Geometry: final body of the model. Coordinates: model frame, mm. A direction names the side the tool comes from. Give positions to 0.01 mm unless a question says otherwise; leave off trailing zeros. Order: outer loops, then holes, each group sorted by start corner. A loop starts at its lowest first (then second) coordinate and runs counter-clockwise, first axis right, second up. Notation, with made-up numbers: (40.5, -29) -> (69.5, -29) arc R11 cw to (69.5, -9) -> close; hole circle Ø1 at (38, -12). An arc over 180 degrees is marked (long way). One line per question, with ' | ' between items.
from build123d import *

# Parameters (mm, degrees)
SKETCH1_W             = 241.3
SKETCH1_H             = 50.8
BOSS_EXTRUDE1_DEPTH   = 12.7
SKETCH3_R             = 4
CUT_EXTRUDE1_DEPTH    = 124.947055229
CUT_EXTRUDE2_DEPTH    = 124.947055229
F_8_CLEARANCE_HOLE1_D = 4.4958
SKETCH10_R            = 1.905
CUT_EXTRUDE3_DEPTH    = 5.08
BOSS_EXTRUDE2_DEPTH   = 12.7
CUT_EXTRUDE4_DEPTH    = 124.947055239
SKETCH14_R            = 1.27
CUT_EXTRUDE5_DEPTH    = 6.35
SKETCH15_W            = 7.607640742
SKETCH15_H            = 9.409671306
CUT_EXTRUDE6_DEPTH    = 124.947055239
SKETCH16_W            = 0.104572849
SKETCH16_H            = 0.14582332
CUT_EXTRUDE8_DEPTH    = 124.947055239
SKETCH18_R            = 2.0828
CUT_EXTRUDE9_DEPTH    = 132.523201385
LPATTERN1_COUNT       = 3
LPATTERN1_PITCH       = 10.16


with BuildPart() as part:
    # Sketch1 → Boss-Extrude1 (new body)
    with BuildSketch(Plane.XY):
        Rectangle(SKETCH1_W, SKETCH1_H)
    extrude(amount=BOSS_EXTRUDE1_DEPTH)

    # Sketch3 → Cut-Extrude1 (cut, through all)
    with BuildSketch(Plane.XY.offset(12.7)):
        with Locations((-107.95, 0)):
            Circle(SKETCH3_R)
    extrude(amount=-CUT_EXTRUDE1_DEPTH, mode=Mode.SUBTRACT)

    # Sketch5 → Cut-Extrude2 (cut, through all)
    with BuildSketch(Plane.XY.offset(12.7)):
        with BuildLine():
            Line((-59.990308431, -25.4), (-105.894198974, -6.008009832))
            Line((-105.894198974, -6.008009832), (-109.958209517, -6.024084539))
            Line((-109.958209517, -6.024084539), (-118.086209517, -6.024084539))
            Line((-118.086209517, -6.024084539), (-118.086209517, 2.230915461))
            Line((-118.086209517, 2.230915461), (-113.895209517, 2.230915461))
            ThreePointArc((-113.895209517, 2.230915461), (-111.566364668, 5.219617475), (-107.95, 6.35))
            Line((-107.95, 6.35), (-67.015128773, 25.4))
            Line((-67.015128773, 25.4), (-120.65, 25.4))
            Line((-120.65, 25.4), (-120.65, -25.4))
            Line((-120.65, -25.4), (-59.990308431, -25.4))
        make_face()
        with BuildLine():
            Line((120.65, -25.4), (120.65, 25.4))
            ThreePointArc((120.65, 25.4), (72.371753541, -10.785174559), (13.834903468, -25.4))
            Line((13.834903468, -25.4), (120.65, -25.4))
        make_face()
    extrude(amount=-CUT_EXTRUDE2_DEPTH, mode=Mode.SUBTRACT)

    # #8 Clearance Hole1 (through all)
    with Locations(Plane(origin=(0, 0, 0), x_dir=(-1, 0, 0), z_dir=(0, 0, -1))):
        with Locations((44.020428639, 16.052306877), (44.020428639, -2.997693123)):
            f_8_clearance_hole1 = Hole(F_8_CLEARANCE_HOLE1_D / 2)

    # Sketch10 → Cut-Extrude3 (cut)
    with BuildSketch(Plane.ZY.offset(114.3)):
        with Locations((6.089367744, 0)):
            Circle(SKETCH10_R)
    extrude(amount=-CUT_EXTRUDE3_DEPTH, mode=Mode.SUBTRACT)

    # Sketch11 → Boss-Extrude2 (add)
    with BuildSketch(Plane.XY.offset(12.7)):
        Polygon((-93.824923554, 12.923434781), (-109.445923554, 5.653836977), (-109.445923554, 11.556774368), align=None)
    extrude(amount=-BOSS_EXTRUDE2_DEPTH)

    # Sketch12 → Cut-Extrude4 (cut, through all)
    with BuildSketch(Plane.XY.offset(12.7)):
        with BuildLine():
            Line((10.021655843, 16.51), (-33.573281826, 16.51))
            Line((-33.573281826, 16.51), (-33.573281826, -16.51))
            Line((-33.573281826, -16.51), (13.63000586, -16.51))
            ThreePointArc((13.63000586, -16.51), (23.12933387, -15.748429471), (32.557173193, -14.358081305))
            Line((32.557173193, -14.358081305), (10.021655843, 16.51))
        make_face()
        with BuildLine():
            Line((26.733875346, 16.51), (46.823064271, -11.007216822))
            ThreePointArc((46.823064271, -11.007216822), (74.177600846, 0.070720235), (98.687628211, 16.51))
            Line((98.687628211, 16.51), (26.733875346, 16.51))
        make_face()
    extrude(amount=-CUT_EXTRUDE4_DEPTH, mode=Mode.SUBTRACT)

    # Sketch14 → Cut-Extrude5 (cut)
    with BuildSketch(Plane(origin=(0.022106899, -5.589070571, 0), x_dir=(0.9999921775754317, 0.003955349282477503, 0), z_dir=(0.003955349282477503, -0.9999921775754317, 0))):
        with Locations((-107.949155569, 6.35)):
            Circle(SKETCH14_R)
    extrude(amount=-CUT_EXTRUDE5_DEPTH, mode=Mode.SUBTRACT)

    # Sketch15 → Cut-Extrude6 (cut, through all)
    with BuildSketch(Plane.XY.offset(12.7)):
        with Locations((113.836536756, 17.520164347)):
            Rectangle(SKETCH15_W, SKETCH15_H)
    extrude(amount=-CUT_EXTRUDE6_DEPTH, mode=Mode.SUBTRACT)

    # Sketch16 → Cut-Extrude8 (cut, through all)
    with BuildSketch(Plane.XY.offset(12.7)):
        with Locations((117.692643551, 22.15208834)):
            Rectangle(SKETCH16_W, SKETCH16_H)
    extrude(amount=-CUT_EXTRUDE8_DEPTH, mode=Mode.SUBTRACT)

    # Sketch18 → Cut-Extrude9 (cut, through all)
    with BuildSketch(Plane(origin=(0, 25.4, 0), x_dir=(1, 0, 0), z_dir=(0, 1, 0))):
        with Locations(Location((114.3, -6.35, 0), (0, 0, 180))):
            Circle(SKETCH18_R)
    extrude(amount=-CUT_EXTRUDE9_DEPTH, mode=Mode.SUBTRACT)

    # LPattern1: #8 Clearance Hole1 ×3
    with Locations(*[(-i * LPATTERN1_PITCH, 0, 0) for i in range(1, LPATTERN1_COUNT)]):
        add(f_8_clearance_hole1, mode=Mode.SUBTRACT)


solid = part.part
1) Section C-C on x = -69.5. Return loops of the section in (y, z).
Check result:
outline: (-21.38, 0) -> (24.24, 0) -> (24.24, 12.7) -> (-21.38, 12.7) -> close
2) Section A-A on x = 114.3. Return loops of the section in (y, z) (3 decimals), plus the area to 3 significant figures.
Check result:
outline: (22.225, 0) -> (25.4, 0) -> (25.4, 4.267) -> (22.225, 4.267) -> close; (22.225, 8.433) -> (25.4, 8.433) -> (25.4, 12.7) -> (22.225, 12.7) -> close | area: 27.1 mm^2
3) Set-up query: faces 5 (the flat face through (110.033, 18, 6)), 6 (the flat face through (36.64, 2.94, 6.44)), 7 (the flat face through (-109.446, 9, 6)). Return all of +Z, -Z, +X, -X, +Y, -Y with unobstructed straight access to the full face (end or side cutting, diameter ignored); none if empty.
Check result:
face 5: +Z, -Z, +X, -Y | face 6: +Z, -Z | face 7: +Z, -Z, -X, +Y
4) Contact query for flat-ended pins moving along their axis: pin 1 Ø4.5 at (x, z) = (-116.5, 7.5) entering from +Y; pin 2 Ø6.5 at (x, z) = (-115, 5.5) entering from -Y; pin 3 Ø1.6 at (y, z) = (9, 6) entering from -X. Output: stop coordinate, or through.
Check result:
pin 1: stops at y = 2.23 | pin 2: stops at y = -6.02 | pin 3: stops at x = -109.45
5) Material intervals for probe 1 along X at (y, z) = (14.5, 3.25); probe 2 along Y at (x, z) = (32, 3.25); probe 3 along X at (y, z) = (11.5, 8), sorted ascending. Write a range as from..to.
Check result:
probe 1: x = -90.44..-65.97, -62.71..-55.81, -52.55..-45.65, -42.39..-33.57, 11.49..28.2, 96.22..109.9 | probe 2: y = -23.48..-14.46, -13.59..9.3, 16.51..25.4 | probe 3: x = -109.45..-33.57, 13.68..30.39, 92.31..106.53
6) Pull-direction query (X, two-part tool) for faces 1 (the cylindrical face through (22.997, -15.763, 6.439)), 2 (the flat face through (21.447, 0.86, 6.439)), 3 (the flat face through (3, 17, 0)), 4 (the cylindrical face through (-112.192, 4.725, 6.439)); classes: +X half, -X half, draft (parallel to the pull), parting line (faces both ways), or undercut.
Check result:
face 1: undercut | face 2: undercut | face 3: draft | face 4: -X half
7) Section B-B on z = 2. Count the separate pieces of the cut face and the enclosed holes in it, plus the area to 3 significant figures.
Check result:
separate pieces: 1 | enclosed holes: 9 | area: 6,020 mm^2
